Source: CAD feature listing. Evaluate the final solid. Frame: model axes, mm. Give positions to 0.01 mm unless a question says otherwise; leave off trailing zeros. Order: outer loops, then holes, each group sorted by start corner. A loop starts at its lowest first (then second) coordinate and runs counter-clockwise, first axis right, second up. Notation, with made-up numbers: M -36,-36.75 L -30,-36.75 A23 ccw -30,-19.75 Z; hole C -39.5,65.25 d2. An arc over 180 degrees is marked long. Answer as a JSON object with one key per item and string values. Group by question number.
1. Material intervals for L1, parallel to X at y = -7.75, z = 29.05; L2, parallel to Z at x = -49.2, y = -4; L3, parallel to X at y = -8.5, z = 28.75, sorted ascending. Write a range as [from, to].
2. Section query A-A (y = -14.25). Output: boundary loops of the cut face in (x, z).
3. Section query C-C (z = 26.3). Output: boundary loops of the cut face in (x, y).
4. Section query B-B (x = -46.15). Output: boundary loops of the cut face in (y, z), plus the area to 3 significant figures.
5. Pin query (flat end, axial travel): P1, Ø1.5, axis at x = -46, y = -11.5, coming from the +Z side; P2, Ø1, axis at y = -13.5, z = 28.5, coming from the -X side. Return the tip coordinate at first contact, or that it passes through.
from build123d import *

# Parameters (mm, degrees)
F0_R     = 2
F1_DEPTH = 63
F2_DEPTH = 50
F3_DEPTH = 15
F4_DEPTH = 10
F5_DEPTH = 1
F6_DEPTH = 1
F7_DEPTH = 5
F8_DEPTH = 3


with BuildPart() as f1:
    # F0 (on Front) → F1 (new body)
    with BuildSketch(Plane.XZ):
        with Locations((-47.7000027895, 27.4500008672)):
            Circle(F0_R)
    extrude(amount=F1_DEPTH)

    # F2 (cut): a face of the model
    f2_faces = [f1.faces().sort_by_distance(p)[0] for p in [
        (-47.7000027895, -63, 27.4500008672),
    ]]
    extrude(f2_faces, amount=-F2_DEPTH, mode=Mode.SUBTRACT)

    # F3 (add): a face of the model
    f3_faces = [f1.faces().sort_by_distance(p)[0] for p in [
        (-47.7000027895, -13, 27.4500008672),
    ]]
    extrude(f3_faces, amount=F3_DEPTH)

    # F4 (cut): a face of the model
    f4_faces = [f1.faces().sort_by_distance(p)[0] for p in [
        (-47.7000027895, -28, 27.4500008672),
    ]]
    extrude(f4_faces, amount=-F4_DEPTH, mode=Mode.SUBTRACT)

    # F5 (cut): a face of the model
    f5_faces = [f1.faces().sort_by_distance(p)[0] for p in [
        (-47.7000027895, -18, 27.4500008672),
    ]]
    extrude(f5_faces, amount=-F5_DEPTH, mode=Mode.SUBTRACT)

    # F6 (cut): a face of the model
    f6_faces = [f1.faces().sort_by_distance(p)[0] for p in [
        (-47.7000027895, -17, 27.4500008672),
    ]]
    extrude(f6_faces, amount=-F6_DEPTH, mode=Mode.SUBTRACT)

    # F7 (add): a face of the model
    f7_faces = [f1.faces().sort_by_distance(p)[0] for p in [
        (-47.7000027895, -16, 27.4500008672),
    ]]
    extrude(f7_faces, amount=F7_DEPTH)

    # F8 (cut): a face of the model
    f8_faces = [f1.faces().sort_by_distance(p)[0] for p in [
        (-47.7000027895, -21, 27.4500008672),
    ]]
    extrude(f8_faces, amount=-F8_DEPTH, mode=Mode.SUBTRACT)


solid = f1.part
Answer sheet:
{
 "1": {"L1": "[-48.9, -46.5]", "L2": "[26.13, 28.77]", "L3": "[-49.22, -46.18]"},
 "2": {"outline": "C -47.7,27.45 d4"},
 "3": {"outline": "M -49.34,-18 L -46.06,-18 L -46.06,0 L -49.34,0 Z"},
 "4": {"outline": "M -18,26.19 L 0,26.19 L 0,28.71 L -18,28.71 Z", "area": "45.5 mm^2"},
 "5": {"P1": "z = 29.21", "P2": "x = -49.62"}
}
